Geometry check sheet. Reference: the model listing, model coordinates, mm. Coordinates: 2 decimals unless noted, no trailing zeros. Loops run counter-clockwise (first coordinate to the right, second up) from the corner with the lowest first, then second, coordinate; pieces in that order, holes last. Notation, with made-up numbers: (72, 47) - (124, 47) arc R4 cw to (124, 51) - close; hole circle Ø3 at (61, -7). An arc over 180 degrees is marked (long way). One line per item, written item: value.
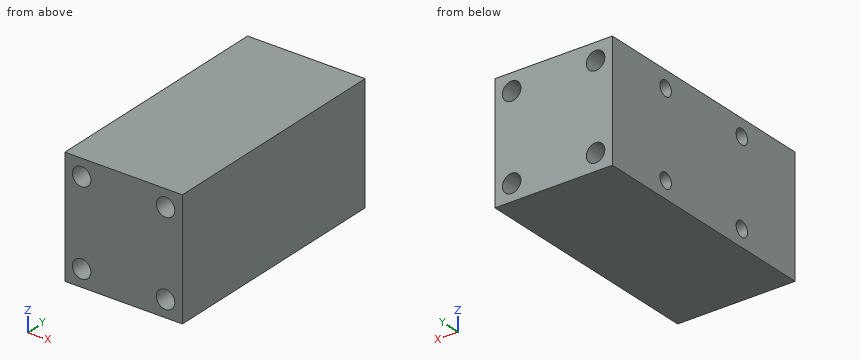
from build123d import *

# Parameters (mm, degrees)
SKETCH1_W           = 35
SKETCH1_H           = 72
BOSS_EXTRUDE1_DEPTH = 17.5


with BuildPart() as part:
    # Sketch1 → Boss-Extrude1 (new, symmetric)
    with BuildSketch(Plane.XY):
        Rectangle(SKETCH1_W, SKETCH1_H)
    extrude(amount=BOSS_EXTRUDE1_DEPTH, both=True)

    # Sketch3 → M5 Clearance Hole1 (revolve, cut)
    with BuildSketch(Plane(origin=(-12.5, 36, -12.5), x_dir=(0, 0, 1), z_dir=(1, 0, 0))):
        Polygon((0, 0), (0, 9.652366702), (2.75, 8), (2.75, 0), align=None)
    m5_clearance_hole1 = revolve(axis=Axis((-12.5, 42.35, -12.5), (0, -1, 0)), mode=Mode.SUBTRACT)

    # Mirror1: M5 Clearance Hole1 across plane
    add(m5_clearance_hole1.mirror(Plane(origin=(0, 0, 0), x_dir=(0, 0, 1), z_dir=(1, 0, 0))), mode=Mode.SUBTRACT)

    # Mirror2: M5 Clearance Hole1 across plane
    add(m5_clearance_hole1.mirror(Plane.XY), mode=Mode.SUBTRACT)

    # Mirror2 copy 1 sketch → Mirror2 copy 1 (revolve, cut)
    with BuildSketch(Plane(origin=(12.5, 36, 12.5), x_dir=(0, 0, -1), z_dir=(-1, 0, 0))):
        Polygon((0, 0), (0, 9.652366702), (2.75, 8), (2.75, 0), align=None)
    revolve(axis=Axis((12.5, 42.35, 12.5), (0, -1, 0)), mode=Mode.SUBTRACT)

    # Mirror3: M5 Clearance Hole1 across plane
    add(m5_clearance_hole1.mirror(Plane.ZX), mode=Mode.SUBTRACT)

    # Mirror3 copy 1 sketch → Mirror3 copy 1 (revolve, cut)
    with BuildSketch(Plane(origin=(12.5, -36, -12.5), x_dir=(0, 0, 1), z_dir=(-1, 0, 0))):
        Polygon((0, 0), (0, 9.652366702), (2.75, 8), (2.75, 0), align=None)
    revolve(axis=Axis((12.5, -42.35, -12.5), (0, 1, 0)), mode=Mode.SUBTRACT)

    # Mirror3 copy 2 sketch → Mirror3 copy 2 (revolve, cut)
    with BuildSketch(Plane(origin=(-12.5, -36, 12.5), x_dir=(0, 0, -1), z_dir=(1, 0, 0))):
        Polygon((0, 0), (0, 9.652366702), (2.75, 8), (2.75, 0), align=None)
    revolve(axis=Axis((-12.5, -42.35, 12.5), (0, 1, 0)), mode=Mode.SUBTRACT)

    # Mirror3 copy 3 sketch → Mirror3 copy 3 (revolve, cut)
    with BuildSketch(Plane(origin=(12.5, -36, 12.5), x_dir=(0, 0, -1), z_dir=(-1, 0, 0))):
        Polygon((0, 0), (0, -9.652366702), (2.75, -8), (2.75, 0), align=None)
    revolve(axis=Axis((12.5, -42.35, 12.5), (0, -1, 0)), mode=Mode.SUBTRACT)

    # Sketch6 → M4 Clearance Hole1 (revolve, cut)
    with BuildSketch(Plane(origin=(-17.5, 15, -12.5), x_dir=(0, 0, 1), z_dir=(0, 1, 0))):
        Polygon((0, 0), (0, 9.351936393), (2.25, 8), (2.25, 0), align=None)
    m4_clearance_hole1 = revolve(axis=Axis((-23.85, 15, -12.5), (1, 0, 0)), mode=Mode.SUBTRACT)

    # Mirror4: M4 Clearance Hole1 across plane
    add(m4_clearance_hole1.mirror(Plane.XY), mode=Mode.SUBTRACT)

    # Mirror5: M4 Clearance Hole1 across plane
    add(m4_clearance_hole1.mirror(Plane.ZX), mode=Mode.SUBTRACT)

    # Mirror5 copy 1 sketch → Mirror5 copy 1 (revolve, cut)
    with BuildSketch(Plane(origin=(-17.5, -15, 12.5), x_dir=(0, 0, -1), z_dir=(0, -1, 0))):
        Polygon((0, 0), (0, 9.351936393), (2.25, 8), (2.25, 0), align=None)
    revolve(axis=Axis((-23.85, -15, 12.5), (1, 0, 0)), mode=Mode.SUBTRACT)


solid = part.part
(1) Cross-section at A-A on y = 31.5. Record the cut outline in (x, z).
Reply:
outline: (-17.5, -17.5) - (17.5, -17.5) - (17.5, 17.5) - (-17.5, 17.5) - close; hole circle Ø5.5 at (-12.5, -12.5); hole circle Ø5.5 at (-12.5, 12.5); hole circle Ø5.5 at (12.5, -12.5); hole circle Ø5.5 at (12.5, 12.5)
(2) Material ranges on probe 1 along X at (y, z) = (33.5, 12.5); probe 2 along Z at (x, y) = (-12.25, 15), recorded low to high. Write a range as from..to.
Reply:
probe 1: -17.5..-15.25, -9.75..9.75, 15.25..17.5
probe 2: -17.5..-14.75, -10.25..10.25, 14.75..17.5
(3) Go/stop test with flat-tipped pins: pin 1 Ø5 at (x, z) = (-12.5, 12.5) entering from -Y; pin 2 Ø5 at (x, z) = (12.5, 12.5) entering from +Y; pin 3 Ø3.5 at (x, z) = (-12.5, -12.5) entering from +Y. Record where each tip stops, or that it passes through.
Reply:
pin 1: y = -27.85
pin 2: y = 27.85
pin 3: y = 27.4
